CAD build for the part. Positions are in the model's coordinates, mm. A direction names the side the tool comes from. Round coordinates to 2 decimals unless told otherwise and drop trailing zeros. Write each loop counter-clockwise with the first axis right and the second up, starting at its lowest first coordinate (ties: lowest second). Pieces come first, ordered by that corner, then holes. Notation, with made-up numbers: (-1, 3) - (21, 3) arc R11 ccw to (21, 9) - close; hole circle Ø8 at (46, 62.25). An arc over 180 degrees is marked (long way). Put each result on its own line as item: value. Start each with the question number.
Item 1: Cut at C-C (z = 25.5). Give the cut face in (x, y).
Item 2: Cut at B-B (x = 2). Give the cut face in (y, z), and give its area (3 significant figures).
Item 3: Pin check, flat tips, straight feed: pin 1 Ø13.5 at (x, z) = (13, 29) entering from +Y; pin 2 Ø5 at (x, z) = (3, 29.5) entering from -Y; pin 3 Ø10 at (y, z) = (16.5, 26.5) entering from +X. Stop position of each tip, or through.
Item 4: Cut at D-D (y = 6). Give the cut face in (x, z).
Item 5: 3-axis set-ups, long thin cutter, end or side, ignore diameter. For faces 5 (the flat face through (2.889, -19, 25)), 6 (the flat face through (6, 19, 20.526)), 7 (the flat face through (1, -25.4, 25)): which of +Z, -Z, +X, -X, +Y, -Y reach the whole face in a straight line?
Item 6: Mould opens along Z. For faces 1 (the flat face through (9.239, 19, 25)), 2 (the flat face through (6, -32, 18.304)), 3 (the flat face through (9.239, -19, 25)), 4 (the flat face through (5, 38.1, 6)) say: released by +Z, released by -Z, zero draft, split by the parting line, or undercut.
Item 7: Cut at A-A (y = -22). Give the cut face in (x, z).
Item 8: Drill centre lines: line 1 (Y direction, x = -8, z = 28); line 2 (Z direction, x = 19.5, y = -26); line 3 (X direction, y = 20.5, z = 28). Where is each one in solid material? Low to high. Write a range as from..to.
```python
from build123d import *

# Parameters (mm, degrees)
F1_DEPTH = 38.1
F2_DEPTH = 25.4
F3_DEPTH = 12.7


with BuildPart() as f1:
    # F0 (on Front) → F1 (new body, symmetric)
    with BuildSketch(Plane.XZ):
        Polygon((7.498131, 18.303821), (-11.430653, 18.303821), (-11.430653, -5.979048), (22.280489, -5.979048), (22.280489, 18.303821), (14.65952, 18.303821), align=None)
    extrude(amount=F1_DEPTH, both=True)

    # F0 (on Front) → F2 (join, symmetric)
    with BuildSketch(Plane.XZ):
        Polygon((7.498131, 20.526321), (7.498131, 18.303821), (14.65952, 18.303821), (14.65952, 20.526321), (9.238502, 20.526321), align=None)
        with BuildLine():
            ThreePointArc((3.028655, 34.988191), (-7.312834, 29.34284), (-11.430653, 18.303821))
            Line((-11.430653, 18.303821), (7.498131, 18.303821))
            Line((7.498131, 18.303821), (7.498131, 20.526321))
            Line((7.498131, 20.526321), (2.888502, 20.526321))
            Line((2.888502, 20.526321), (2.888502, 29.416321))
            Line((2.888502, 29.416321), (9.238502, 29.416321))
            Line((9.238502, 29.416321), (9.238502, 20.526321))
            Line((9.238502, 20.526321), (14.65952, 20.526321))
            Line((14.65952, 20.526321), (14.65952, 18.303821))
            Line((14.65952, 18.303821), (22.280489, 18.303821))
            ThreePointArc((22.280489, 18.303821), (16.463937, 31.041573), (3.028655, 34.988191))
        make_face()
    extrude(amount=F2_DEPTH, both=True)

    # F0 (on Front) → F3 (join, symmetric)
    with BuildSketch(Plane.XZ):
        Polygon((2.888502, 20.526321), (7.498131, 20.526321), (9.238502, 20.526321), (9.238502, 29.416321), (2.888502, 29.416321), align=None)
    extrude(amount=F3_DEPTH, both=True)


solid = f1.part
```
Output values:
1. outline: (-9.82, -25.4) - (2.89, -25.4) - (2.89, -12.7) - (9.24, -12.7) - (9.24, -25.4) - (20.67, -25.4) - (20.67, 25.4) - (9.24, 25.4) - (9.24, 12.7) - (2.89, 12.7) - (2.89, 25.4) - (-9.82, 25.4) - close
2. outline: (-38.1, -5.98) - (38.1, -5.98) - (38.1, 18.3) - (25.4, 18.3) - (25.4, 34.81) - (-25.4, 34.81) - (-25.4, 18.3) - (-38.1, 18.3) - close
2. area: 2,690 mm2
3. pin 1: y = 25.4
3. pin 2: y = -25.4
3. pin 3: x = 21.97
4. outline: (-11.43, -5.98) - (22.28, -5.98) - (22.28, 18.3) arc R16.86 ccw to (3.03, 34.99) arc R16.86 ccw to (-11.43, 18.3) - close
5. face 5: -Y
5. face 6: +Y
5. face 7: +Z, +X, -X, -Y
6. face 1: undercut
6. face 2: released by +Z
6. face 3: undercut
6. face 4: zero draft
7. outline: (-11.43, -5.98) - (22.28, -5.98) - (22.28, 18.3) arc R16.86 ccw to (3.03, 34.99) arc R16.86 ccw to (-11.43, 18.3) - close; hole (2.89, 20.53) - (9.24, 20.53) - (9.24, 29.42) - (2.89, 29.42) - close
8. line 1: -25.4..25.4
8. line 2: -5.98..18.3
8. line 3: -8.36..2.89, 9.24..19.21
